```python
from build123d import *

# Parameters (mm, degrees)
SKETCH1_W           = 30
SKETCH1_H           = 25
BOSS_EXTRUDE1_DEPTH = 45
SKETCH2_W           = 5
SKETCH2_H           = 5
CUT_EXTRUDE1_DEPTH  = 45
SKETCH4_R           = 2
CUT_EXTRUDE17_DEPTH = 9
SKETCH5_W           = 9
SKETCH5_H           = 13
CUT_EXTRUDE18_DEPTH = 56.509008278
CUT_EXTRUDE19_START = -9
SKETCH6_R           = 2
CUT_EXTRUDE19_DEPTH = 9
SKETCH7_R           = 6
CUT_EXTRUDE20_DEPTH = 50.053542176


with BuildPart() as part:
    # Sketch1 → Boss-Extrude1 (new body)
    with BuildSketch(Plane(origin=(0, 0, 0), x_dir=(1, 0, 0), z_dir=(0, 1, 0))):
        Rectangle(SKETCH1_W, SKETCH1_H)
    extrude(amount=BOSS_EXTRUDE1_DEPTH)

    # Sketch2 → Cut-Extrude1 (cut)
    with BuildSketch(Plane(origin=(0, 45, 0), x_dir=(1, 0, 0), z_dir=(0, 1, 0))):
        with Locations((12.5, 0)):
            Rectangle(SKETCH2_W, SKETCH2_H)
        with Locations((-12.5, 0)):
            Rectangle(SKETCH2_W, SKETCH2_H)
    extrude(amount=-CUT_EXTRUDE1_DEPTH, mode=Mode.SUBTRACT)

    # Sketch4 → Cut-Extrude17 (cut)
    with BuildSketch(Plane(origin=(0, 0, -12.5), x_dir=(-1, 0, 0), z_dir=(0, 0, -1))):
        with Locations((8, 4)):
            Circle(SKETCH4_R)
        with Locations((-8, 4)):
            Circle(SKETCH4_R)
    extrude(amount=-CUT_EXTRUDE17_DEPTH, mode=Mode.SUBTRACT)

    # Sketch5 → Cut-Extrude18 (cut, through all)
    with BuildSketch(Plane.ZY.offset(15)):
        with Locations((0, 6.5)):
            Rectangle(SKETCH5_W, SKETCH5_H)
    extrude(amount=-CUT_EXTRUDE18_DEPTH, mode=Mode.SUBTRACT)

    # Sketch6 → Cut-Extrude19 (cut)
    with BuildSketch(Plane.XY.offset(12.5).offset(CUT_EXTRUDE19_START)):
        with Locations(Location((8, 4, 0), (0, 0, 180))):
            Circle(SKETCH6_R)
        with Locations(Location((-8, 4, 0), (0, 0, 180))):
            Circle(SKETCH6_R)
    extrude(amount=CUT_EXTRUDE19_DEPTH, mode=Mode.SUBTRACT)

    # Sketch7 → Cut-Extrude20 (cut, through all)
    with BuildSketch(Plane(origin=(0, 45, 0), x_dir=(1, 0, 0), z_dir=(0, 1, 0))):
        with Locations(Location((0, 0, 0), (0, 0, 270))):
            Circle(SKETCH7_R)
    extrude(amount=-CUT_EXTRUDE20_DEPTH, mode=Mode.SUBTRACT)


solid = part.part
```
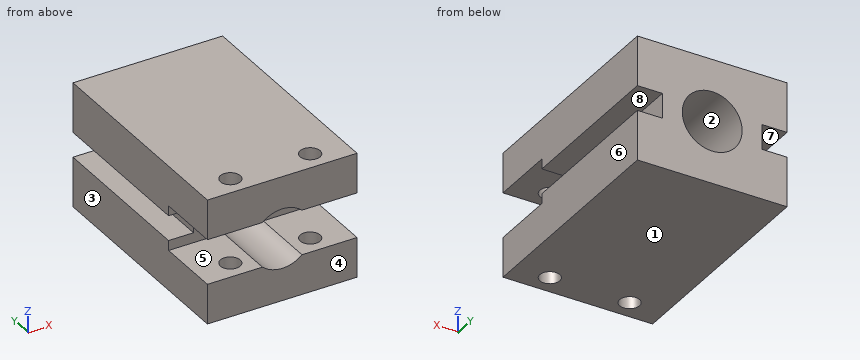
Geometry: final body of the model. Coordinates: model frame, mm. Face numbers are marked on the shaded views. A direction names the side the tool comes from. Coordinates: 2 decimals unless noted, no trailing zeros. Order: outer loops, then holes, each group sorted by start corner. A loop starts at its lowest first (then second) coordinate and runs counter-clockwise, first axis right, second up. Notation, with made-up numbers: (14, 72.5) - (60, 72.5) arc R17 ccw to (60, 91.5) - close; hole circle Ø11 at (-22.75, 78). An arc over 180 degrees is marked (long way). Return JSON: item names as keys, results as strings. Group by question number.
1. Pin query (flat end, axial travel): pin 1 (1.5 mm diameter, centred on y = 22, z = 0, fed in from -X); pin 2 (4 mm diameter, centred on x = 7.5, z = -0.5, fed in from -Y). Return the tip coordinate at first contact, or that it passes through.
2. Pull-direction query (X, two-part tool) for the marked faces 1, 2 and 3; classes: pulls with the +X half, pulls with the -X half, needs draft (parallel to the pull), parting line crosses it, or undercut.
3. Cut plane B-B (y = 38.5). Output: boundary loops of the cut face in (x, z), plus the area to 3 significant figures.
4. Set-up query: the marked faces 4, 5, 6, 7 and 8. Return all of +Z, -Z, +X, -X, +Y, -Y with unobstructed straight access to the full face (end or side cutting, diameter ignored); none if empty.
5. Cut plane A-A (x = 8). Output: boundary loops of the cut face in (y, z), plus the area to 3 significant figures.
6. Cut plane C-C (z = 0). Output: boundary loops of the cut face in (x, y).
7. Material intervals for line 1 along X through (y, z) = (4, 8.5); line 2 along Z through (x, y) = (10.75, 5.5); line 3 along Y through (x, z) = (-8, -10.5), sorted ascending. Write a range as [from, to].
8. Cut plane D-D (y = 4). Output: boundary loops of the cut face in (x, z), plus the area to 3 significant figures.
Resolved:
{
 "1": {"pin 1": "stops at x = -10", "pin 2": "stops at y = 13"},
 "2": {"face 1": "needs draft", "face 2": "undercut", "face 3": "pulls with the -X half"},
 "3": {"outline": "(-15, -12.5) - (15, -12.5) - (15, -2.5) - (10, -2.5) - (10, 2.5) - (15, 2.5) - (15, 12.5) - (-15, 12.5) - (-15, 2.5) - (-10, 2.5) - (-10, -2.5) - (-15, -2.5) - close; hole circle Ø12 at (0, 0)", "area": "587 mm²"},
 "4": {"face 4": "+Z, -Z, +X, -X, -Y", "face 5": "+X, -X, -Y", "face 6": "+Z, -Z, +X, +Y, -Y", "face 7": "-X, +Y, -Y", "face 8": "+X, +Y, -Y"},
 "5": {"outline": "(0, -12.5) - (2, -12.5) - (2, -4.5) - (0, -4.5) - close; (0, 4.5) - (2, 4.5) - (2, 12.5) - (0, 12.5) - close; (6, -12.5) - (45, -12.5) - (45, 12.5) - (6, 12.5) - (6, 4.5) - (13, 4.5) - (13, -4.5) - (6, -4.5) - close", "area": "944 mm²"},
 "6": {"outline": "(-10, 13) - (-6, 13) - (-6, 45) - (-10, 45) - close; (6, 13) - (10, 13) - (10, 45) - (6, 45) - close"},
 "7": {"line 1": "x = [-15, -10], [-6, 6], [10, 15]", "line 2": "z = [-12.5, -4.5], [4.5, 12.5]", "line 3": "y = [0, 2], [6, 45]"},
 "8": {"outline": "(-15, -12.5) - (-10, -12.5) - (-10, -4.5) - (-15, -4.5) - close; (-15, 4.5) - (-10, 4.5) - (-10, 12.5) - (-15, 12.5) - close; (-6, -12.5) - (6, -12.5) - (6, -4.5) - (3.97, -4.5) arc R6 cw to (-3.97, -4.5) - (-6, -4.5) - close; (-6, 4.5) - (-3.97, 4.5) arc R6 cw to (3.97, 4.5) - (6, 4.5) - (6, 12.5) - (-6, 12.5) - close; (10, -12.5) - (15, -12.5) - (15, -4.5) - (10, -4.5) - close; (10, 4.5) - (15, 4.5) - (15, 12.5) - (10, 12.5) - close", "area": "336 mm²"}
}
